Design review of the part built by this model. Coordinates are the model's own, in mm. Face numbers are marked on the shaded views. A direction names the side the tool comes from. Round coordinates to 2 decimals unless told otherwise and drop trailing zeros. Loops run counter-clockwise (first coordinate to the right, second up) from the corner with the lowest first, then second, coordinate; pieces in that order, holes last. Notation, with made-up numbers: M 29,18.5 L 53,18.5 A25 cw 53,54.5 Z; hole C 20,3 d1. An arc over 180 degrees is marked long. Answer as CSV lines item,"result". Start each with the question number.
from build123d import *

# Parameters (mm, degrees)
SKIZZE1_W                            = 48
SKIZZE1_H                            = 25
SKIZZE1_R                            = 8.25
SKIZZE1_R_2                          = 1.5
AUFSATZ_LINEAR_AUSTRAGEN1_DEPTH      = 2
SKIZZE2_W                            = 48
SKIZZE2_H                            = 5
AUFSATZ_LINEAR_AUSTRAGEN2_DEPTH      = 2
SKIZZE3_W                            = 48
SKIZZE3_H                            = 22
AUFSATZ_LINEAR_AUSTRAGEN3_DEPTH      = 2
AUFSATZ_LINEAR_AUSTRAGEN4_DEPTH      = 1.5
SCHNITT_LINEAR_AUSTRAGEN1_DEPTH      = 56.702642494
SCHNITT_LINEAR_AUSTRAGEN1_DEPTH_BACK = 56.702642494
SKIZZE6_W                            = 13
SKIZZE6_H                            = 6
SCHNITT_LINEAR_AUSTRAGEN2_DEPTH      = 56.702642494
SCHNITT_LINEAR_AUSTRAGEN2_DEPTH_BACK = 56.702642494
SKIZZE7_R                            = 1.2
FASE1_SIZE                           = 5.5
FASE1_SIZE_2                         = 2.001836288


with BuildPart() as part:
    # Skizze1 → Aufsatz-Linear austragen1 (new body)
    with BuildSketch(Plane(origin=(0, 23.26672716, 0), x_dir=(1, 0, 0), z_dir=(0, 1, 0))):
        with Locations((18.159741318, -23.319374593)):
            Rectangle(SKIZZE1_W, SKIZZE1_H)
        with Locations(Location((5.436155106, -22.674374593, 0), (0, 0, 90))):
            Circle(SKIZZE1_R, mode=Mode.SUBTRACT)
        with Locations(Location((30.746155106, -22.674374593, 0), (0, 0, 90))):
            Circle(SKIZZE1_R, mode=Mode.SUBTRACT)
        with Locations(Location((39.346155106, -31.529374593, 0), (0, 0, 90))):
            Circle(SKIZZE1_R_2, mode=Mode.SUBTRACT)
        with Locations(Location((39.346155106, -13.819374593, 0), (0, 0, 90))):
            Circle(SKIZZE1_R_2, mode=Mode.SUBTRACT)
        with Locations(Location((-3.163844894, -13.819374593, 0), (0, 0, 90))):
            Circle(SKIZZE1_R_2, mode=Mode.SUBTRACT)
        with Locations(Location((-3.163844894, -31.529374593, 0), (0, 0, 90))):
            Circle(SKIZZE1_R_2, mode=Mode.SUBTRACT)
        with BuildLine():
            Line((21.271155106, -29.094374598), (14.911155106, -29.094374598))
            ThreePointArc((14.911155106, -29.094374598), (11.911155106, -32.094374598), (14.911155106, -35.094374598))
            Line((14.911155106, -35.094374598), (21.271155106, -35.094374598))
            ThreePointArc((21.271155106, -35.094374598), (24.271155106, -32.094374598), (21.271155106, -29.094374598))
        make_face(mode=Mode.SUBTRACT)
        with BuildLine():
            Line((14.911155106, -11.544374589), (21.271155106, -11.544374589))
            ThreePointArc((21.271155106, -11.544374589), (24.271155106, -14.544374589), (21.271155106, -17.544374589))
            Line((21.271155106, -17.544374589), (14.911155106, -17.544374589))
            ThreePointArc((14.911155106, -17.544374589), (11.911155106, -14.544374589), (14.911155106, -11.544374589))
        make_face(mode=Mode.SUBTRACT)
    extrude(amount=-AUFSATZ_LINEAR_AUSTRAGEN1_DEPTH)

    # Skizze2 → Aufsatz-Linear austragen2 (add)
    with BuildSketch(Plane(origin=(0, 21.26672716, 0), x_dir=(-1, 0, 0), z_dir=(0, -1, 0))):
        with Locations((-18.159741318, -38.319374593)):
            Rectangle(SKIZZE2_W, SKIZZE2_H)
    extrude(amount=-AUFSATZ_LINEAR_AUSTRAGEN2_DEPTH)

    # Skizze3 → Aufsatz-Linear austragen3 (add)
    with BuildSketch(Plane.XY.offset(40.819374593)):
        with Locations((18.159741318, 10.26672716)):
            Rectangle(SKIZZE3_W, SKIZZE3_H)
    extrude(amount=-AUFSATZ_LINEAR_AUSTRAGEN3_DEPTH)

    # Skizze5 → Aufsatz-Linear austragen4 (add, symmetric)
    with BuildSketch(Plane(origin=(32.159741318, 0, 0), x_dir=(0, 0, -1), z_dir=(1, 0, 0))):
        Polygon((-38.819374593, 17.26672716), (-38.819374593, 21.26672716), (-34.819374593, 21.26672716), align=None)
    aufsatz_linear_austragen4 = extrude(amount=AUFSATZ_LINEAR_AUSTRAGEN4_DEPTH, both=True)

    # Spiegeln1: Aufsatz-Linear austragen4 across plane
    add(aufsatz_linear_austragen4.mirror(Plane(origin=(18.159741318, 0, 0), x_dir=(0, 0, 1), z_dir=(1, 0, 0))))

    # Skizze6 → Schnitt-Linear austragen1 (cut, two sides: drawn at the far end of the back side and taken through both)
    with BuildSketch(Plane(origin=(0, 0, 38.819374593), x_dir=(-1, 0, 0), z_dir=(0, 0, -1)).offset(-SCHNITT_LINEAR_AUSTRAGEN1_DEPTH_BACK)):
        with Locations((-18.159741318, 14.26672716)):
            Rectangle(SKIZZE6_W, SKIZZE6_H)
    extrude(amount=SCHNITT_LINEAR_AUSTRAGEN1_DEPTH + SCHNITT_LINEAR_AUSTRAGEN1_DEPTH_BACK, mode=Mode.SUBTRACT)

    # Skizze7 → Schnitt-Linear austragen2 (cut, two sides: drawn at the far end of the back side and taken through both)
    with BuildSketch(Plane(origin=(0, 0, 38.819374593), x_dir=(-1, 0, 0), z_dir=(0, 0, -1)).offset(-SCHNITT_LINEAR_AUSTRAGEN2_DEPTH_BACK)):
        with Locations((-36.159741318, 11.26672716)):
            Circle(SKIZZE7_R)
        with Locations(Location((-0.159741318, 11.26672716, 0), (0, 0, 180))):
            Circle(SKIZZE7_R)
    extrude(amount=SCHNITT_LINEAR_AUSTRAGEN2_DEPTH + SCHNITT_LINEAR_AUSTRAGEN2_DEPTH_BACK, mode=Mode.SUBTRACT)

    # Fase1
    # the kernel refuses this chamfer: 5.5, 2.001836288 mm, written as the material it takes off along each edge
    with BuildSketch(Plane(origin=(-20.108329711, -0.73327284, 38.819374593), x_dir=(0, 0.9999130865277315, -0.013184058198645307), z_dir=(1, 0, 0))) as fase1_piece_1:
        Polygon((FASE1_SIZE * 0.999913086528, FASE1_SIZE * 0.0131840581986), (-FASE1_SIZE_2 * 0.0131840582017, FASE1_SIZE_2 * 0.99991308676), (0, 0), align=None)
    extrude(amount=76.536142058, mode=Mode.SUBTRACT)


solid = part.part
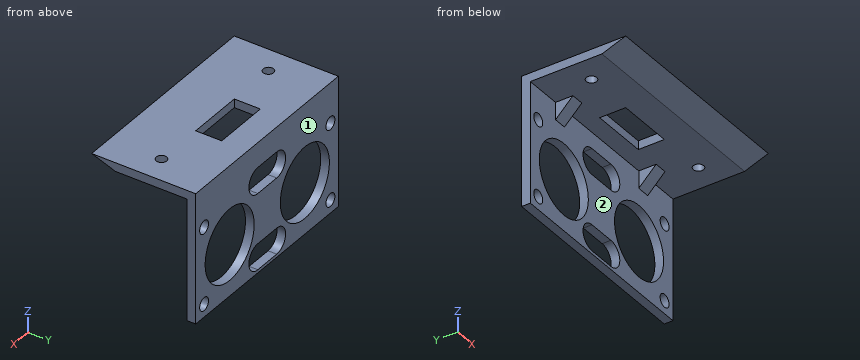
Item 1: To check wall thickness, follow line 1 (Z direction, x = 5.5, y = 22.25); line 2 (Y direction, x = 22.5, z = 36.75); line 3 (Z direction, x = 3, y = 18.25). State the ranges of each line that lie inside material, in increasing order.
Item 2: Insertion check: pin 1 Ø2 at (x, z) = (24, 27) entering from -Y; pin 2 Ø4.5 at (y, z) = (18.5, 36) entering from -X; pin 3 Ø2.5 at (x, z) = (-3.16, 31.53) entering from -Y; pin 4 Ø2 at (y, z) = (19.5, 36) entering from +X. Each pin has a flat end and moves straight along its axis. Give the tip position at first contact, or say it passes through.
Item 3: Consider section D-D, the plane x = 4. Write out the cut boundary in (y, z), then the cut area to 3 significant figures.
Item 4: Consider section C-C, the plane z = 17. Write out the cut boundary in (x, y), then the cut area to 3 significant figures.
Item 5: Tool access review of the marked faces 1 and 2: name each direction out of +Z, -Z, +X, -X, +Y, -Y from which nothing blocks a thin tool from reaching the whole face with its end or side.
Item 6: Consider section B-B, the plane y = 13. Write out the cut boundary in (x, z).
Item 7: Consider section A-A, the plane x = 17.5. Write out the cut boundary in (y, z), then the cut area to 3 significant figures.
Found:
1,line 1,"z = 10.82 to 14.42, 30.92 to 40.82"
1,line 2,"y = 21.27 to 23.27"
1,line 3,"z = 37.84 to 40.82"
2,pin 1,"stops at y = 21.27"
2,pin 2,"stops at x = 2.66"
2,pin 3,"passes through"
2,pin 4,"stops at x = 33.66"
3,outline,"M -0.73,40.82 L 4.77,38.82 L 17.27,38.82 L 21.27,34.82 L 21.27,30.8 L 23.27,30.8 L 23.27,40.82 Z; M 21.27,10.82 L 23.27,10.82 L 23.27,14.55 L 21.27,14.55 Z"
3,area,"74.0 mm^2"
4,outline,"M -5.84,21.27 L -0.55,21.27 L -0.55,23.27 L -5.84,23.27 Z; M 11.42,21.27 L 13.19,21.27 L 13.19,23.27 L 11.42,23.27 Z; M 22.99,21.27 L 24.76,21.27 L 24.76,23.27 L 22.99,23.27 Z; M 36.73,21.27 L 42.16,21.27 L 42.16,23.27 L 36.73,23.27 Z"
4,area,"28.5 mm^2"
5,face 1,"+Z, -Z, +X, -X, +Y"
5,face 2,"-Z, -Y"
6,outline,"M -5.84,38.82 L 11.66,38.82 L 11.66,40.82 L -5.84,40.82 Z; M 24.66,38.82 L 42.16,38.82 L 42.16,40.82 L 24.66,40.82 Z"
7,outline,"M -0.73,40.82 L 4.77,38.82 L 11.27,38.82 L 11.27,40.82 Z; M 17.27,38.82 L 21.27,38.82 L 21.27,35.09 L 23.27,35.09 L 23.27,40.82 L 17.27,40.82 Z; M 21.27,10.82 L 23.27,10.82 L 23.27,11.54 L 21.27,11.54 Z; M 21.27,17.54 L 23.27,17.54 L 23.27,29.09 L 21.27,29.09 Z"
7,area,"62.5 mm^2"
